For this review, take the finished solid that the model builds, in its own axes (mm). A direction names the side the tool comes from. Give positions to 0.01 mm unless a question says otherwise; leave off trailing zeros. Write each loop counter-clockwise with the first axis right and the second up, starting at its lowest first coordinate (ties: lowest second). Pieces come first, ordered by that corner, then holes.
1) Machinability: for faces 5 (the face through (55.48, 2.46, -11.17)), 6 (the face through (61.421, 79, -12)), 7 (the face through (54.03, 87.48, -10.17)), 8 (the face through (22.84, 85.12, -0.99)), 9 (the face through (-13.579, 79, -12)), which of the approach directions +Z, -Z, +X, -X, +Y, -Y give a long, thin tool a straight path to every point of the face, cutting with its end or side? Answer none if there is none.
2) For P1, Ø3, axis at x = -10.08, z = -11.72, coming from the -Y side; P2, Ø8, axis at y = 12, z = -10.5, coming from the +X side; P3, Ø8, axis at x = 23.92, y = 90, coming from the -Z side; P4, Ø8, axis at y = 85, z = -10.5, coming from the -X side, all flat-tipped, find the tip position at first contact; note any pin that passes through.
3) We need section A-A on y = 90. Give the boundary of the cut face in (x, z), and give its area (3 significant figures).
4) We need section D-D on y = 66.5. Give the boundary of the cut face in (x, z), and give its area (3 significant figures).
5) We need section B-B on z = -17. Give the boundary of the cut face in (x, y).
6) Draft analysis for pull direction Z (two halves, no side actions). For faces 1 (the face through (26, 88, -2)), 2 (the face through (54.03, 27.48, -10.17)), 3 (the face through (-5.97, 82.52, -10.17)), 4 (the face through (63.921, 79, -2)), state which applies: pulls with the +Z half, pulls with the -Z half, needs draft (parallel to the pull), parting line crosses it, or undercut.
7) We need section C-C on y = 25. Give the boundary of the cut face in (x, z), and give its area (3 significant figures).
8) Wall thickness on line 1 along Y through (x, z) = (2, -8.25); line 2 along Z through (x, y) = (-7.25, 145); line 3 along X through (y, z) = (13.5, -2.5): over which ranges is each line inside the solid? List them lowest first.
from build123d import *
from OCP.BRepAlgoAPI import BRepAlgoAPI_Cut
from OCP.TopTools import TopTools_ListOfShape

# Parameters (mm, degrees)
BOSS_EXTRUDE1_DEPTH = 160
SKETCH2_R           = 5
CUT_EXTRUDE1_DEPTH  = 2
SKETCH3_R           = 2.5
CUT_EXTRUDE2_DEPTH  = 174.084103307
SKETCH4_R           = 2.5
SKETCH4_R_2         = 6
CUT_EXTRUDE3_DEPTH  = 174.286199049
SKETCH5_R           = 2.5
CUT_EXTRUDE4_DEPTH  = 5
SKETCH6_R           = 2.5
SKETCH6_R_2         = 4.5
CUT_EXTRUDE5_DEPTH  = 15
CUT_EXTRUDE6_START  = -15
SKETCH7_R           = 2.5
SKETCH7_R_2         = 3.51695151
CUT_EXTRUDE6_DEPTH  = 15


with BuildPart() as part:
    # Sketch1 → Boss-Extrude1 (new body)
    with BuildSketch(Plane(origin=(0, 0, 0), x_dir=(1, 0, 0), z_dir=(0, 1, 0))):
        Polygon((-16.079290349, -9.231e-06), (63.920709651, -9.231e-06), (63.920709651, 4.999990769), (61.420709651, 4.999990769), (61.420709651, 18.499990769), (-13.579290349, 18.499990769), (-13.579290349, 4.999990769), (-16.079290349, 4.999990769), align=None)
    extrude(amount=BOSS_EXTRUDE1_DEPTH)


with BuildPart() as cut_extrude1_tool:
    # Sketch2 → Cut-Extrude1 (new body)
    with BuildSketch(Plane.XY):
        with Locations((23.920709651, 90)):
            Circle(SKETCH2_R)
    extrude(amount=-CUT_EXTRUDE1_DEPTH)


with BuildPart() as part_1:
    add(part.part)

    # Cut-Extrude1: cut by cut_extrude1_tool, with a tolerance
    cut_extrude1_stock = TopTools_ListOfShape()
    cut_extrude1_stock.Append(part_1.part.wrapped)
    cut_extrude1_tools = TopTools_ListOfShape()
    cut_extrude1_tools.Append(cut_extrude1_tool.part.wrapped)
    cut_extrude1_cut = BRepAlgoAPI_Cut()
    cut_extrude1_cut.SetArguments(cut_extrude1_stock)
    cut_extrude1_cut.SetTools(cut_extrude1_tools)
    cut_extrude1_cut.SetFuzzyValue(0.00001)
    cut_extrude1_cut.Build()
    add(Compound.cast(cut_extrude1_cut.Shape()).solids(), mode=Mode.REPLACE)

    # Sketch3 → Cut-Extrude2 (cut, through all)
    with BuildSketch(Plane.XY.offset(-2)):
        with Locations((23.920709651, 90)):
            Circle(SKETCH3_R)
    extrude(amount=-CUT_EXTRUDE2_DEPTH, mode=Mode.SUBTRACT)


with BuildPart() as cut_extrude3_tool:
    # Sketch4 → Cut-Extrude3 (new, through all)
    with BuildSketch(Plane.XY):
        with BuildLine():
            ThreePointArc((8.920709651, 52), (-1.321931036, 56.242640687), (2.920709651, 46))
            Line((2.920709651, 46), (2.920709651, 52))
            Line((2.920709651, 52), (8.920709651, 52))
        make_face()
        with BuildLine():
            Line((2.920709651, 52), (2.920709651, 46))
            ThreePointArc((2.920709651, 46), (7.163350338, 47.757359313), (8.920709651, 52))
            Line((8.920709651, 52), (2.920709651, 52))
        make_face()
        with Locations((44.920709651, 52)):
            Circle(SKETCH4_R)
        with Locations((2.920709651, 12)):
            Circle(SKETCH4_R)
        with Locations((44.920709651, 12)):
            Circle(SKETCH4_R_2)
    extrude(amount=-CUT_EXTRUDE3_DEPTH)


with BuildPart() as part_2:
    add(part_1.part)

    # Cut-Extrude3: cut by cut_extrude3_tool, with a tolerance
    cut_extrude3_stock = TopTools_ListOfShape()
    cut_extrude3_stock.Append(part_2.part.wrapped)
    cut_extrude3_tools = TopTools_ListOfShape()
    cut_extrude3_tools.Append(cut_extrude3_tool.part.wrapped)
    cut_extrude3_cut = BRepAlgoAPI_Cut()
    cut_extrude3_cut.SetArguments(cut_extrude3_stock)
    cut_extrude3_cut.SetTools(cut_extrude3_tools)
    cut_extrude3_cut.SetFuzzyValue(0.00001)
    cut_extrude3_cut.Build()
    add(Compound.cast(cut_extrude3_cut.Shape()).solids(), mode=Mode.REPLACE)

    # Sketch5 → Cut-Extrude4 (cut)
    with BuildSketch(Plane.XZ):
        with Locations(Location((57.920709651, -11.71640591, 0), (0, 0, 270))):
            Circle(SKETCH5_R)
        with Locations(Location((-10.079290349, -11.71640591, 0), (0, 0, 270))):
            Circle(SKETCH5_R)
    extrude(amount=-CUT_EXTRUDE4_DEPTH, mode=Mode.SUBTRACT)

    # Sketch6 → Cut-Extrude5 (cut)
    with BuildSketch(Plane(origin=(61.420709651, 0, 0), x_dir=(0, 0, -1), z_dir=(1, 0, 0))):
        with Locations((10.499990769, 145)):
            Circle(SKETCH6_R)
        with Locations((10.499990769, 85)):
            Circle(SKETCH6_R)
        with Locations((10.499990769, 25)):
            Circle(SKETCH6_R)
        with Locations((10.499990769, 12)):
            Circle(SKETCH6_R_2)
    extrude(amount=-CUT_EXTRUDE5_DEPTH, mode=Mode.SUBTRACT)

    # Sketch7 → Cut-Extrude6 (cut)
    with BuildSketch(Plane.ZY.offset(13.579290349).offset(CUT_EXTRUDE6_START)):
        with Locations(Location((-10.499990769, 145, 0), (0, 0, 180))):
            Circle(SKETCH7_R)
        with Locations(Location((-10.499990769, 85, 0), (0, 0, 180))):
            Circle(SKETCH7_R)
        with Locations(Location((-10.499990769, 25, 0), (0, 0, 180))):
            Circle(SKETCH7_R)
        with Locations((-10.499990769, 52)):
            Circle(SKETCH7_R_2)
    extrude(amount=CUT_EXTRUDE6_DEPTH, mode=Mode.SUBTRACT)


solid = part_2.part
Results list:
1. face 5: -Y
1. face 6: -Z, +X, +Y, -Y
1. face 7: +X
1. face 8: +Z
1. face 9: -Z, -X, +Y, -Y
2. P1: stops at y = 5
2. P2: stops at x = 40.45
2. P3: stops at z = -18.5
2. P4: stops at x = -13.58
3. outline: (-16.08, -5) - (-13.58, -5) - (-13.58, -18.5) - (21.42, -18.5) - (21.42, -2) - (18.92, -2) - (18.92, 0) - (-16.08, 0) - close; (26.42, -18.5) - (61.42, -18.5) - (61.42, -5) - (63.92, -5) - (63.92, 0) - (28.92, 0) - (28.92, -2) - (26.42, -2) - close
3. area: 1,310 mm2
4. outline: (-16.08, -5) - (-13.58, -5) - (-13.58, -18.5) - (61.42, -18.5) - (61.42, -5) - (63.92, -5) - (63.92, 0) - (-16.08, 0) - close
4. area: 1,410 mm2
5. outline: (-13.58, 0) - (61.42, 0) - (61.42, 160) - (-13.58, 160) - close; hole circle Ø12 at (2.92, 52); hole circle Ø5 at (2.92, 12); hole circle Ø5 at (23.92, 90); hole circle Ø12 at (44.92, 12); hole circle Ø5 at (44.92, 52)
6. face 1: pulls with the +Z half
6. face 2: undercut
6. face 3: undercut
6. face 4: needs draft
7. outline: (-16.08, -5) - (-13.58, -5) - (-13.58, -8) - (1.42, -8) - (1.42, -13) - (-13.58, -13) - (-13.58, -18.5) - (61.42, -18.5) - (61.42, -13) - (46.42, -13) - (46.42, -8) - (61.42, -8) - (61.42, -5) - (63.92, -5) - (63.92, 0) - (-16.08, 0) - close
7. area: 1,260 mm2
8. line 1: y = 0 to 9.68, 14.32 to 46.07, 57.93 to 160
8. line 2: z = -18.5 to -13, -8 to 0
8. line 3: x = -16.08 to 0.92, 4.92 to 39.11, 50.73 to 63.92
